Verification items for the finished model (mm, model axes). A direction names the side the tool comes from. Round coordinates to 2 decimals unless told otherwise and drop trailing zeros. Order: outer loops, then holes, each group sorted by start corner. A loop starts at its lowest first (then second) coordinate and runs counter-clockwise, first axis right, second up. Notation, with made-up numbers: M 43.25,8.25 L 77.25,8.25 A14 ccw 77.25,26.25 Z; hole C 60.5,-1 d7. An arc over 180 degrees is marked long. Return JSON: item names as keys, results as strings. Group by question number.
from build123d import *

# Parameters (mm, degrees)
BOSS_EXTRUDE1_DEPTH = 4
SKETCH2_W           = 33
SKETCH2_H           = 20
SKETCH2_W_2         = 10
SKETCH2_H_2         = 10
CUT_EXTRUDE1_DEPTH  = 5
CUT_EXTRUDE2_DEPTH  = 10
SKETCH4_R           = 3
CUT_EXTRUDE3_DEPTH  = 10


with BuildPart() as part:
    # Sketch1 → Boss-Extrude1 (new body)
    with BuildSketch(Plane.XY):
        Polygon((27, -31), (27, -35), (7, -35), (7, -31), (-42, -31), (-42, 31), (42, 31), (42, -31), align=None)
    extrude(amount=BOSS_EXTRUDE1_DEPTH)

    # Sketch2 → Cut-Extrude1 (cut)
    with BuildSketch(Plane(origin=(0, 0, 0), x_dir=(-1, 0, 0), z_dir=(0, 0, -1))):
        with Locations((25.5, -21)):
            Rectangle(SKETCH2_W, SKETCH2_H)
        with Locations((-37, 26)):
            Rectangle(SKETCH2_W_2, SKETCH2_H_2)
    extrude(amount=-CUT_EXTRUDE1_DEPTH, mode=Mode.SUBTRACT)

    # Sketch3 → Cut-Extrude2 (cut)
    with BuildSketch(Plane(origin=(0, 0, 0), x_dir=(-1, 0, 0), z_dir=(0, 0, -1))):
        Polygon((32, 22.6), (32, 12.6), (27.6, 12.6), (27.6, 22.6), (26.1, 22.6), (26.1, 26), (27.6, 26), (27.6, 31), (32, 31), (32, 26), (33.5, 26), (33.5, 22.6), align=None)
        Polygon((-17.6, 22.6), (-17.6, 12.6), (-22, 12.6), (-22, 22.6), (-23.5, 22.6), (-23.5, 26), (-22, 26), (-22, 31), (-17.6, 31), (-17.6, 26), (-16.1, 26), (-16.1, 22.6), align=None)
    extrude(amount=-CUT_EXTRUDE2_DEPTH, mode=Mode.SUBTRACT)

    # Sketch4 → Cut-Extrude3 (cut)
    with BuildSketch(Plane(origin=(0, 0, 0), x_dir=(-1, 0, 0), z_dir=(0, 0, -1))):
        with Locations((30, 8)):
            Circle(SKETCH4_R)
        with Locations((-19.5, 8)):
            Circle(SKETCH4_R)
    extrude(amount=-CUT_EXTRUDE3_DEPTH, mode=Mode.SUBTRACT)


solid = part.part
1. Go/stop test with flat-tipped pins: pin 1 (2 mm diameter, centred on x = 38, z = 2.5, fed in from -Y); pin 2 (12 mm diameter, centred on x = 4, y = -25.5, fed in from -Z); pin 3 (1.2 mm diameter, centred on y = 27.5, z = 2.5, fed in from +X); pin 4 (1.2 mm diameter, centred on x = -32.5, z = 1.5, fed in from -Y). Record where each tip stops, or that it passes through.
2. Access from +Z, -Z, +X, -X, +Y, -Y to the whole of each face (thin tool, end or side, straight path). Record for faces 1 (the face through (-9, -21, 2)), 2 (the face through (23.5, 24, 2)), 3 (the face through (32, 26, 2)), 4 (the face through (-30, 12.6, 2)).
3. Cross-section at B-B (y = 8). Enter the section's corners in (x, z).
4. Thickness scan on line 1 along X through (y, z) = (17, 3.7); line 2 along X through (y, z) = (28.5, 3.7); line 3 along Y through (x, z) = (19.5, 2.45). Record the ranges inside material, lowest first. Write a range as from..to.
5. Cross-section at C-C (z = 1.7). Give the number of separate pieces and of enclosed holes in the cut face, plus the area to 3 significant figures.
6. Cross-section at D-D (x = -30). Enter the section's corners in (y, z).
7. Draft check along X on faces 5 (the face through (-27.6, 28, 2)), 6 (the face through (27, 31, 2)), 7 (the face through (27, -33, 2)). Enter one of: +X half, -X half, draft (parallel to the pull), parting line (faces both ways), or undercut.
8. Cross-section at A-A (x = 19.5). Enter the section's corners in (y, z).
Computed:
{
 "1": {"pin 1": "stops at y = -31", "pin 2": "stops at z = 0", "pin 3": "stops at x = 32", "pin 4": "stops at y = -11"},
 "2": {"face 1": "+Z, -Z, -X, -Y", "face 2": "+Z, -Z", "face 3": "+Z, -Z, +X, +Y", "face 4": "+Z, -Z, +Y"},
 "3": {"outline": "M -42,0 L -33,0 L -33,4 L -42,4 Z; M -27,0 L 16.5,0 L 16.5,4 L -27,4 Z; M 22.5,0 L 42,0 L 42,4 L 22.5,4 Z"},
 "4": {"line 1": "x = -42..-32, -27.6..17.6, 22..42", "line 2": "x = -42..-32, -27.6..17.6, 22..32", "line 3": "y = -35..5, 11..12.6"},
 "5": {"separate pieces": "1", "enclosed holes": "2", "area": "4,290 mm²"},
 "6": {"outline": "M -11,0 L 5,0 L 5,4 L -11,4 Z; M 11,0 L 12.6,0 L 12.6,4 L 11,4 Z"},
 "7": {"face 5": "undercut", "face 6": "draft", "face 7": "+X half"},
 "8": {"outline": "M -35,0 L 5,0 L 5,4 L -35,4 Z; M 11,0 L 12.6,0 L 12.6,4 L 11,4 Z"}
}
